Input: part model. Units: mm. Frame: model coordinates. A direction names the side the tool comes from. Round coordinates to 2 decimals unless told otherwise and drop trailing zeros. Order: outer loops, then holes, each group sorted by start corner. A loop starts at its lowest first (then second) coordinate and runs counter-clockwise, first axis right, second up. Notation, with made-up numbers: M 65.25,-23 L 121.25,-23 A17 ccw 121.25,-2 Z; hole C 13,0.5 d2. An arc over 180 degrees is marked long. One line per question, with ' | ' between items.
```python
from build123d import *

# Parameters (mm, degrees)
BOSS_EXTRUDE2_DEPTH = 1.5
SKETCH5_W           = 1.5
SKETCH5_H           = 8
BOSS_EXTRUDE3_DEPTH = 28
CUT_EXTRUDE1_DEPTH  = 28
CHAMFER1_SIZE       = 2


with BuildPart() as part:
    # Sketch4 → Boss-Extrude2 (new body)
    with BuildSketch(Plane.XY):
        Polygon((-21.818181818, -18.75), (35.181818182, -18.75), (35.181818182, -3.75), (-9.272727273, -3.75), (-20.318181818, -10.75), (-21.818181818, -10.75), align=None)
    extrude(amount=BOSS_EXTRUDE2_DEPTH)

    # Sketch5 → Boss-Extrude3 (add)
    with BuildSketch(Plane(origin=(0, 0, 0), x_dir=(-1, 0, 0), z_dir=(0, 0, -1))):
        with Locations((21.068181818, -14.75)):
            Rectangle(SKETCH5_W, SKETCH5_H)
    extrude(amount=BOSS_EXTRUDE3_DEPTH)

    # Sketch6 → Cut-Extrude1 (cut)
    with BuildSketch(Plane.XY.offset(1.5)):
        with BuildLine():
            Line((18.431818182, -6.75), (18.431818182, -15.75))
            ThreePointArc((18.431818182, -15.75), (20.181818182, -17.5), (21.931818182, -15.75))
            Line((21.931818182, -15.75), (21.931818182, -6.75))
            ThreePointArc((21.931818182, -6.75), (20.181818182, -5), (18.431818182, -6.75))
        make_face()
        with BuildLine():
            Line((28.431818182, -6.75), (28.431818182, -15.75))
            ThreePointArc((28.431818182, -15.75), (30.181818182, -17.5), (31.931818182, -15.75))
            Line((31.931818182, -15.75), (31.931818182, -6.75))
            ThreePointArc((31.931818182, -6.75), (30.181818182, -5), (28.431818182, -6.75))
        make_face()
    extrude(amount=-CUT_EXTRUDE1_DEPTH, mode=Mode.SUBTRACT)

    # Chamfer1
    chamfer1_edges = [part.edges().sort_by_distance(p)[0] for p in [
        (35.181818182, -3.75, 0.75),
        (35.181818182, -18.75, 0.75),
    ]]
    chamfer(chamfer1_edges, length=CHAMFER1_SIZE)


solid = part.part
```
Item 1: Mould query, pull axis X, two halves, no side actions, for faces 1 (the flat face through (6, -11, 1.5)), 2 (the cylindrical face through (20.2, -5, 0.8)), 3 (the flat face through (-20.318, -15, -14)). Classes: +X half, -X half, draft (parallel to the pull), parting line (faces both ways), or undercut.
Report:
face 1: draft | face 2: undercut | face 3: +X half
Item 2: First-contact query: pin 1 (4.5 mm diameter, centred on x = 5.5, y = -11.5, fed in from -Z); pin 2 (0.8 mm diameter, centred on y = -9.5, z = 0.5, fed in from -X); pin 3 (0.8 mm diameter, centred on x = -21, z = -7.5, fed in from +Y). Flat tips, straight axial feed; report the tip coordinate or a pass-through.
Report:
pin 1: z = 0 | pin 2: x = -18.98 | pin 3: y = -10.75
Item 3: Section query C-C, the plane y = -8.5. Return loops of the section in (x, z).
Report:
outline: M -16.77,0 L 18.43,0 L 18.43,1.5 L -16.77,1.5 Z; M 21.93,0 L 28.43,0 L 28.43,1.5 L 21.93,1.5 Z; M 31.93,0 L 35.18,0 L 35.18,1.5 L 31.93,1.5 Z
Item 4: Line query: line 1 along Z through (x, y) = (-10.5, -4.75); line 2 along X through (y, z) = (-16.25, -1.5). Output: solid intervals per line, ascending. Write a range as from..to.
Report:
line 1: 0..1.5 | line 2: -21.82..-20.32
Item 5: Section query A-A, the plane y = -13.75. Return loops of the section in (x, z).
Report:
outline: M -21.82,-28 L -20.32,-28 L -20.32,0 L 18.43,0 L 18.43,1.5 L -21.82,1.5 Z; M 21.93,0 L 28.43,0 L 28.43,1.5 L 21.93,1.5 Z; M 31.93,0 L 35.18,0 L 35.18,1.5 L 31.93,1.5 Z
Item 6: Section query B-B, the plane x = 31. Return loops of the section in (y, z), plus the area to 3 significant figures.
Report:
outline: M -18.75,0 L -17.3,0 L -17.3,1.5 L -18.75,1.5 Z; M -5.2,0 L -3.75,0 L -3.75,1.5 L -5.2,1.5 Z | area: 4.36 mm²
Item 7: Section query D-D, the plane z = -21.75. Return loops of the section in (x, y).
Report:
outline: M -21.82,-18.75 L -20.32,-18.75 L -20.32,-10.75 L -21.82,-10.75 Z
Item 8: Access query for faces 4 (the cylindrical face through (20.1, -17.5, 0.8)), 5 (the flat face through (-21, -15, -28)), 6 (the flat face through (7, -11, 0)). Directions: +Z, -Z, +X, -X, +Y, -Y. A direction counts if a zero-diameter tool reaches every point of the face in a straight line with its end or side. Return the directions, or none.
Report:
face 4: +Z, -Z | face 5: -Z, +X, -X, +Y, -Y | face 6: -Z, +X, +Y, -Y
